Verification items for this drawing (mm, ordinates from the low corner). A direction names the side the tool comes from. Round coordinates to 2 decimals unless told otherwise and drop trailing zeros. Write each loop counter-clockwise with the first axis right and the second up, starting at its lowest first coordinate (ties: lowest second). Pieces come first, ordered by that corner, then holes. Notation, with made-up numbers: (80, 7.5) -> (134, 7.5) arc R11 cw to (134, 28.5) -> close; hole circle Ø5 at (33.5, -34.75). An arc over 180 degrees is marked (long way). One line per question, with ' | ' between items.
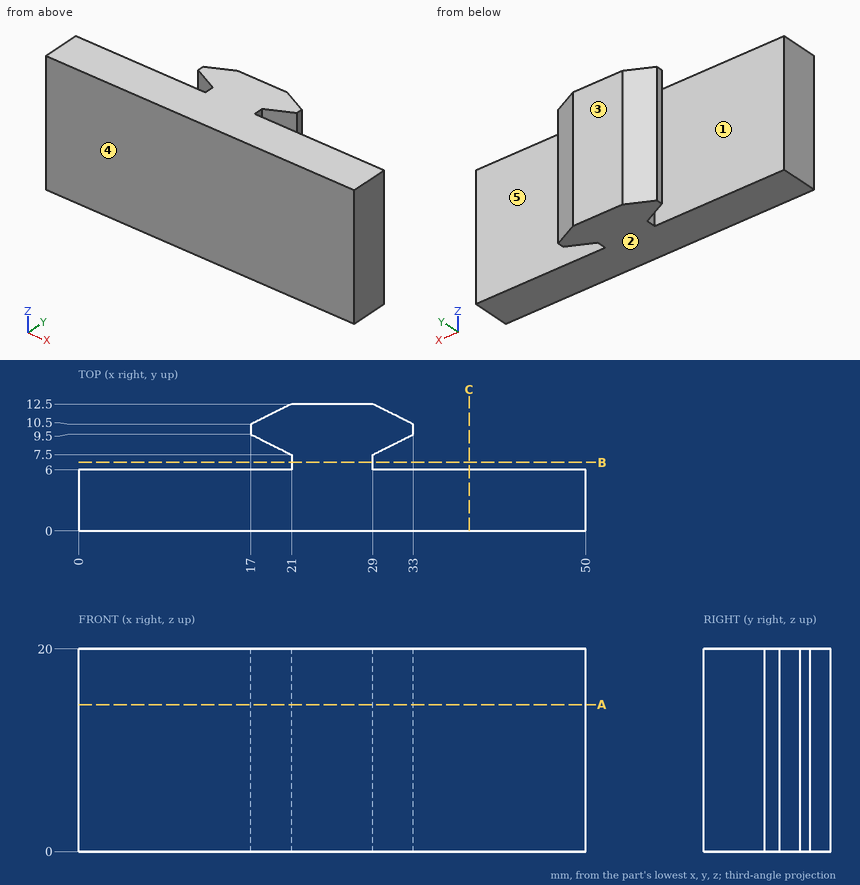
(1) Sectioned sample at C-C on x = 38.5. Record the cut outline in (y, z).
Resolved:
outline: (0, 0) -> (6, 0) -> (6, 20) -> (0, 20) -> close
(2) Draft check along Y on the marked faces 1, 2 and 3. Enter one of: +Y half, -Y half, draft (parallel to the pull), parting line (faces both ways), or undercut.
Resolved:
face 1: undercut | face 2: draft | face 3: +Y half
(3) Material ranges on line 1 (Y direction, x = 36.5, z = 6.5); line 2 (X direction, y = 6.5, z = 8); line 3 (X direction, y = 10, z = 16.75), recorded low to high.
Resolved:
line 1: y = 0 to 6 | line 2: x = 21 to 29 | line 3: x = 17 to 33
(4) Access from +Z, -Z, +X, -X, +Y, -Y to the whole of each face (thin tool, end or side, straight path). Record for the marked faces 4 and 5.
Resolved:
face 4: +Z, -Z, +X, -X, -Y | face 5: +Z, -Z, +X
(5) Sectioned sample at B-B on y = 6.75. Record the cut outline in (x, z), then the cut area to 3 significant figures.
Resolved:
outline: (21, 0) -> (29, 0) -> (29, 20) -> (21, 20) -> close | area: 160 mm2
(6) Sectioned sample at A-A on z = 14.5. Record the cut outline in (x, y).
Resolved:
outline: (0, 0) -> (50, 0) -> (50, 6) -> (29, 6) -> (29, 7.5) -> (33, 9.5) -> (33, 10.5) -> (29, 12.5) -> (21, 12.5) -> (17, 10.5) -> (17, 9.5) -> (21, 7.5) -> (21, 6) -> (0, 6) -> close
(7) Go/stop test with flat-tipped pins: pin 1 (0.5 mm diameter, centred on y = 10, z = 5.5, fed in from -X); pin 2 (1.5 mm diameter, centred on x = 18, z = 11, fed in from +Y) (3 decimals); pin 3 (0.8 mm diameter, centred on y = 6.5, z = 13, fed in from -X). Record where each tip stops, or that it passes through.
Resolved:
pin 1: stops at x = 17 | pin 2: stops at y = 11.375 | pin 3: stops at x = 21
